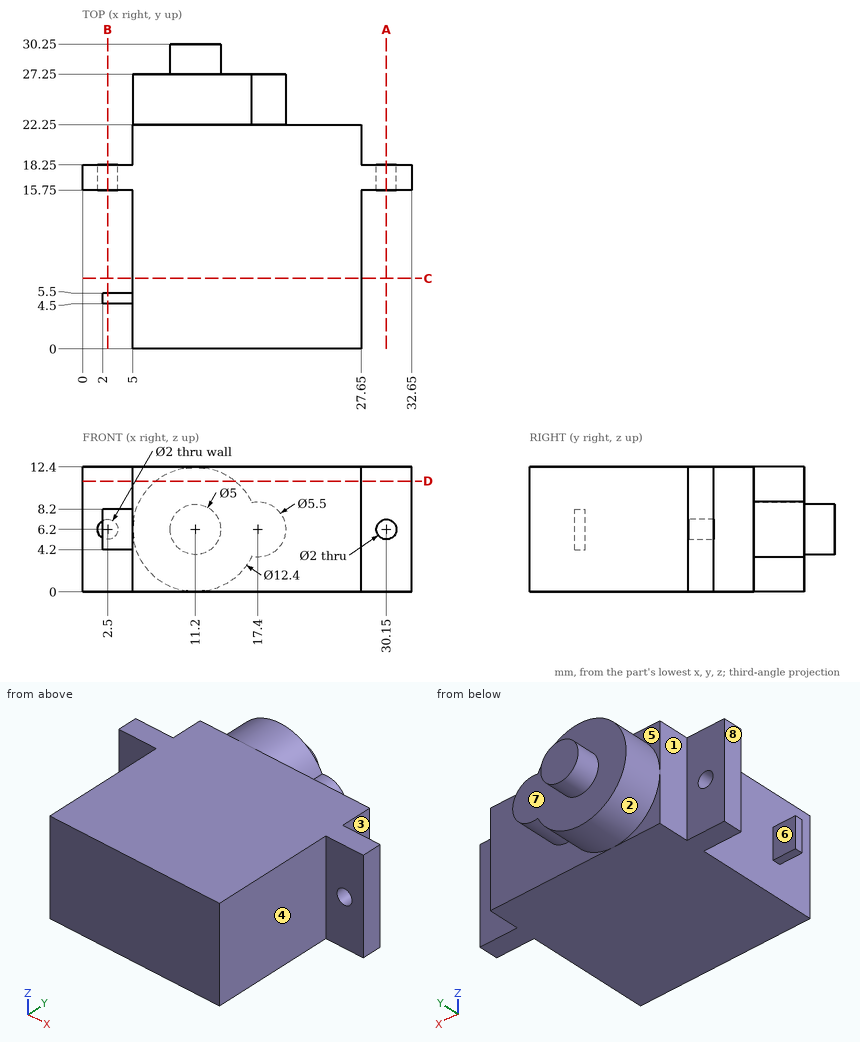
The drawing under review shows one solid part. Ordinate dimensions are in mm from its lowest x, y, z. A direction names the side the tool comes from. Coordinates: 2 decimals unless noted, no trailing zeros. Order: outer loops, then holes, each group sorted by start corner. A loop starts at its lowest first (then second) coordinate and runs counter-clockwise, first axis right, second up. Notation, with made-up numbers: (-6, 20) -> (22, 20) arc R16 ccw to (22, 45) -> close; hole circle Ø8 at (-27, 82). An arc over 180 degrees is marked (long way). Answer as CSV lines item,"result".
Q1. Draft analysis for pull direction Y (two halves, no side actions). For the marked faces 6, 7 and 8, state which applies: released by +Y, released by -Y, zero draft, split by the parting line, or undercut.
Model answer:
face 6,"undercut"
face 7,"released by +Y"
face 8,"zero draft"
Q2. Clearance check with flat-ended pins moving along their axes: pin 1 Ø1.5 at (x, z) = (13, 2) entering from +Y; pin 2 Ø2.5 at (x, z) = (3.5, 6) entering from +Y; pin 3 Ø1.8 at (x, z) = (2.5, 6.2) entering from +Y. State where each tip first meets the part, or that it passes through.
Model answer:
pin 1,"stops at y = 27.25"
pin 2,"stops at y = 18.25"
pin 3,"stops at y = 5.5"
Q3. Wall thickness on line 1 along X through (y, z) = (17.65, 6.2); line 2 along Y through (x, z) = (3, 7.75); line 3 along X through (y, z) = (21, 11.75): over which ranges is each line inside the solid? List them lowest first. Write a range as [from, to].
Model answer:
line 1,"x = [0, 1.5], [3.5, 29.15], [31.15, 32.65]"
line 2,"y = [4.5, 5.5], [15.75, 18.25]"
line 3,"x = [5, 27.65]"
Q4. We need section B-B (x = 2.5). State the section outline as (y, z) points, plus the area to 3 significant figures.
Model answer:
outline,"(4.5, 4.2) -> (5.5, 4.2) -> (5.5, 8.2) -> (4.5, 8.2) -> close; (15.75, 0) -> (18.25, 0) -> (18.25, 5.2) -> (15.75, 5.2) -> close; (15.75, 7.2) -> (18.25, 7.2) -> (18.25, 12.4) -> (15.75, 12.4) -> close"
area,"30.0 mm2"
Q5. We need section A-A (x = 30.15). State the section outline as (y, z) points, plus the area to 3 significant figures.
Model answer:
outline,"(15.75, 0) -> (18.25, 0) -> (18.25, 5.2) -> (15.75, 5.2) -> close; (15.75, 7.2) -> (18.25, 7.2) -> (18.25, 12.4) -> (15.75, 12.4) -> close"
area,"26.0 mm2"
Q6. We need section D-D (z = 11). State the section outline as (x, y) points.
Model answer:
outline,"(0, 15.75) -> (5, 15.75) -> (5, 0) -> (27.65, 0) -> (27.65, 15.75) -> (32.65, 15.75) -> (32.65, 18.25) -> (27.65, 18.25) -> (27.65, 22.25) -> (15.12, 22.25) -> (15.12, 27.25) -> (7.28, 27.25) -> (7.28, 22.25) -> (5, 22.25) -> (5, 18.25) -> (0, 18.25) -> close"
Q7. We need section C-C (y = 7). State the section outline as (x, z) points.
Model answer:
outline,"(5, 0) -> (27.65, 0) -> (27.65, 12.4) -> (5, 12.4) -> close"
Q8. For the marked faces 1, 2, 3, 4 and 5, list the 3-axis set-ups (+Z, -Z, +X, -X, +Y, -Y) from which the entire face can be reached by the end or side of a thin tool; tool diameter is ignored.
Model answer:
face 1,"+Z, -Z, -X, +Y"
face 2,"+Y"
face 3,"+Z, -Z, +X, +Y"
face 4,"+Z, -Z, +X, -Y"
face 5,"+Z, -X, +Y"
